Autodesk Inventor part; units mm, degrees
ref_plane "YZ Plane" through (0, 0, 0) normal (1, 0, 0) x (0, 1, 0)
ref_plane "XZ Plane" through (0, 0, 0) normal (0, 1, 0) x (-1, 0, 0)
ref_plane "XY Plane" through (0, 0, 0) normal (0, 0, 1) x (1, 0, 0)
sketch "Szkic1" plane through (0, 0, 0) normal (0, 1, 0) x (-1, 0, 0)
  line L0 (0, 0) -> (0, -18)
  line L1 (0, -18) -> (-8, -18)
  line L2 (-8, -18) -> (-8, -30)
  line L3 (-8, -30) -> (0, -30)
  line L4 (0, -30) -> (0, -48)
  line L5 (0, -48) -> (-3, -48)
  line L6 (-3, -48) -> (-3, -33)
  line L7 (-3, -33) -> (-11, -33)
  line L8 (-11, -33) -> (-11, -15)
  line L9 (-11, -15) -> (-3, -15)
  line L10 (-3, -15) -> (-3, 0)
  line L11 (-3, 0) -> (0, 0)
  dimension "d0" = 48
  dimension "d2" = 8
  dimension "d3" = 12
  dimension "d4" = 3
  dimension "d5" = 3
  dimension "d6" = 3
extrude "Wyciągnięcie proste1" add sketch "Szkic1" along normal blind 20
fillet "Zaokrąglenie1" radius 2 6 edges at (11, 10, -15) (3, 10, -15) (11, 10, -33) (3, 10, -33) (0, 10, -18) (0, 10, -30)
fillet "Zaokrąglenie2" radius 1 6 edges at (3, 10, 0) (0, 10, 0) (0, 10, -48) (3, 10, -48) (8, 10, -30) (8, 10, -18)
sketch "Szkic2" plane through (0, 0, -32) normal (-1, 0, 0) x (0, 0, 1)
  line L0 (-15, 0) -> (-15, 20)
  line L1 (-15, 0) -> (0, 0)
  line L2 (0, 20) -> (0, 0)
  line L3 (-15, 20) -> (0, 20)
  line L4 (31, 20) -> (31, 0)
  line L5 (16, 20) -> (31, 20)
  line L6 (16, 0) -> (16, 20)
  line L7 (16, 0) -> (31, 0)
  line L8 (15, 0) -> (1, 0)
  line L9 (8, 0) -> (8, 20) construction
  line L10 (3, 20) -> (13, 20)
  circle A0 centre (-9.5, 10) radius 2.6
  circle A1 centre (25.5, 10) radius 2.6
  point P0 (32, 0)
  dimension "d11" = 5.2
  dimension "d13" = 10
  dimension "d14" = 35
extrude "Wyciągnięcie proste2" cut sketch "Szkic2" against normal up to surface (3 mm away) contours A0 | A1
properties part number "motor_clamp_v2"
CAD build for the part. Positions are in the model's coordinates, mm. A direction names the side the tool comes from. Coordinates: 2 decimals unless noted, no trailing zeros. Write each loop counter-clockwise with the first axis right and the second up, starting at its lowest first coordinate (ties: lowest second). Pieces come first, ordered by that corner, then holes. Notation, with made-up numbers: M -34.5,27.25 L -11.5,27.25 A29 ccw -11.5,53.25 Z; hole C 22,52 d8. An arc over 180 degrees is marked long. Answer as a JSON object with one key per item and string values. Group by question number.
1) Saw through at C-C (y = 10). Give the number of separate pieces and of enclosed holes in the cut face, plus the area to 3 significant figures.
2) Tool access for faces 1 (the face through (7, 10, -15)), 2 (the face through (7.699, 10.14, -18.285)), 3 (the face through (0, 10, -38)): list every direction of +Z, -Z, +X, -X, +Y, -Y with a clear straight run to the whole face (end or side of a thin tool).
3) Saw through at B-B (z = -41.5). Write the cut outline in (x, y), plus the area to 3 significant figures.
4) Saw through at D-D (x = 1.5). Write the cut outline in (y, z).
5) Wall check: line 1 (Y direction, x = 2.35, z = -41.5); line 2 (Z direction, x = 7, y = 3); line 3 (X direction, y = 12.5, z = -40). Give the ranges that are in metal, low to high. Write a range as from..to.
6) Pin check, flat tips, straight feed: pin 1 Ø1.5 at (x, y) = (5.5, 10) entering from -Z; pin 2 Ø2.5 at (x, y) = (4.5, 8) entering from +Z; pin 3 Ø6 at (y, z) = (5.5, -25.5) entering from -X. Stop position of each tip, or through.
7) Mould opens along Y. For faces 4 (the face through (1.479, 8.418, -43.563)), 5 (the face through (1.5, 9.9, -48)) say: +Y half, -Y half, draft (parallel to the pull), parting line (faces both ways), or undercut.
8) Saw through at A-A (x = 5.5). Write the cut outline in (y, z), plus the area to 3 significant figures.
Values follow:
{
 "1": {"separate pieces": "3", "enclosed holes": "0", "area": "159 mm2"},
 "2": {"face 1": "+Z, +X, +Y, -Y", "face 2": "-X, +Y, -Y", "face 3": "+Z, -Z, -X, +Y, -Y"},
 "3": {"outline": "M 0,0 L 3,0 L 3,7.4 L 0,7.4 Z; M 0,12.6 L 3,12.6 L 3,20 L 0,20 Z", "area": "44.4 mm2"},
 "4": {"outline": "M 0,-48 L 20,-48 L 20,-30.06 L 0,-30.06 Z; M 0,-17.94 L 20,-17.94 L 20,0 L 0,0 Z; hole C 10,-41.5 d5.2; hole C 10,-6.5 d5.2"},
 "5": {"line 1": "y = 0..7.4, 12.6..20", "line 2": "z = -33..-30, -18..-15", "line 3": "x = 0..3"},
 "6": {"pin 1": "stops at z = -33.02", "pin 2": "stops at z = -13.97", "pin 3": "stops at x = 8"},
 "7": {"face 4": "undercut", "face 5": "draft"},
 "8": {"outline": "M 0,-33 L 20,-33 L 20,-30 L 0,-30 Z; M 0,-18 L 20,-18 L 20,-15 L 0,-15 Z", "area": "120 mm2"}
}
